Read the model definition and answer for the solid it produces. Units are mm, in the model's axes. A direction names the side the tool comes from. Round coordinates to 2 decimals unless told otherwise and drop trailing zeros. Order: outer loops, then holes, each group sorted by start corner. A loop starts at its lowest first (then second) coordinate and runs counter-clockwise, first axis right, second up. Notation, with made-up numbers: (19, 11.25) -> (27, 11.25) arc R14 cw to (27, 19.25) -> close; hole circle Ø10 at (35.5, 2). An arc over 180 degrees is marked (long way). Use a Markdown table: item, result. Add a question column.
1. Section C-C, the plane x = 0 is taken. Give the vertices of the cut face in (y, z), then the cut area to 3 significant figures.
2. Given pin 1 (5.5 mm diameter, centred on x = 0, z = 0, fed in from -Y); pin 2 (2 mm diameter, centred on y = -5.5, z = -2.5, fed in from +X); pin 3 (5 mm diameter, centred on y = -3.5, z = 1, fed in from -X), each flat-ended and moving along its own axis, determine where each tip first touches the part or whether it passes through.
3. For faces 5 (the face through (0, 1.2, 0)), 6 (the face through (9.224, 0.493, -9.331)), 7 (the face through (11.04, 2.46, -10.91)), determine the directions among +Z, -Z, +X, -X, +Y, -Y from which every point of the face is accessible in a straight line to the end or side of a thin tool.
4. Section D-D, the plane x = -11 is taken. Give the vertices of the cut face in (y, z), then the cut area to 3 significant figures.
5. Section A-A, the plane y = 4.25 is taken. Give the vertices of the cut face in (x, z).
6. Section B-B, the plane z = 0 is taken. Give the vertices of the cut face in (x, y), then the cut area to 3 significant figures.
7. Consider L1, parallel to X at y = 0.75, z = -1; L2, parallel to X at y = -5.5, z = 0; L3, parallel to Z at x = 10.5, y = 0.5. Determine where each line is inside the solid, lowest interval first. Write a range as [from, to].
8. The mould has two halves that part along Z. Classify faces 1 (the face through (6, 0, 0)), 2 (the face through (-10.91, 2.46, -11.04)), 3 (the face through (0.1, 0.5, 14.32)), 4 (the face through (0, 2, 15.52)): +Z half, -Z half, draft (parallel to the pull), parting line (faces both ways), or undercut.
```python
from build123d import *

# Parameters (mm, degrees)
EXTRUDE_1_DEPTH     = 5
CUT_EXTRUDE_1_DEPTH = 1
SKETCH_6_R          = 6.15
CUT_EXTRUDE_2_DEPTH = 3.8
SKETCH_8_R          = 4.15
SKETCH_8_R_2        = 3.15
EXTRUDE_4_DEPTH     = 7
SKETCH_9_R          = 5
SKETCH_9_R_2        = 4.15
EXTRUDE_5_DEPTH     = 2


with BuildPart() as part:
    # 스케치1 → 보스-돌출1 (new body)
    with BuildSketch(Plane(origin=(0, 0, 0), x_dir=(1, 0, 0), z_dir=(0, 1, 0))):
        Polygon((15.520132754, 6.428649477), (6.428649477, 15.520132754), (-6.428649477, 15.520132754), (-15.520132754, 6.428649477), (-15.520132754, -6.428649477), (-6.428649477, -15.520132754), (6.428649477, -15.520132754), (15.520132754, -6.428649477), align=None)
        Polygon((5.931593202, 14.320132754), (-5.931593202, 14.320132754), (-14.320132754, 5.931593202), (-14.320132754, -5.931593202), (-5.931593202, -14.320132754), (5.931593202, -14.320132754), (14.320132754, -5.931593202), (14.320132754, 5.931593202), align=None, mode=Mode.SUBTRACT)
        Polygon((14.320132754, 5.931593202), (5.931593202, 14.320132754), (-5.931593202, 14.320132754), (-14.320132754, 5.931593202), (-14.320132754, -5.931593202), (-5.931593202, -14.320132754), (5.931593202, -14.320132754), (14.320132754, -5.931593202), align=None)
    extrude(amount=EXTRUDE_1_DEPTH)

    # 스케치3 → 컷-돌출1 (cut)
    with BuildSketch(Plane.XZ):
        Polygon((5.931593202, -14.320132754), (14.320132754, -5.931593202), (14.320132754, 5.931593202), (5.931593202, 14.320132754), (-5.931593202, 14.320132754), (-14.320132754, 5.931593202), (-14.320132754, -5.931593202), (-5.931593202, -14.320132754), align=None)
        Polygon((5.434536927, -13.120132754), (13.120132754, -5.434536927), (13.120132754, 5.434536927), (5.434536927, 13.120132754), (-5.434536927, 13.120132754), (-13.120132754, 5.434536927), (-13.120132754, -5.434536927), (-5.434536927, -13.120132754), align=None, mode=Mode.SUBTRACT)
    extrude(amount=-CUT_EXTRUDE_1_DEPTH, mode=Mode.SUBTRACT)

    # 스케치6 → 컷-돌출2 (cut)
    with BuildSketch(Plane(origin=(0, 5, 0), x_dir=(1, 0, 0), z_dir=(0, 1, 0))):
        with Locations(Location((0, 0, 0), (0, 0, 270))):
            Circle(SKETCH_6_R)
    extrude(amount=-CUT_EXTRUDE_2_DEPTH, mode=Mode.SUBTRACT)

    # 스케치8 → 보스-돌출4 (add)
    with BuildSketch(Plane.XZ):
        with Locations(Location((0, 0, 0), (0, 0, 90))):
            Circle(SKETCH_8_R)
        with Locations(Location((0, 0, 0), (0, 0, 270))):
            Circle(SKETCH_8_R_2, mode=Mode.SUBTRACT)
    extrude(amount=EXTRUDE_4_DEPTH)

    # 스케치9 → 보스-돌출5 (add)
    with BuildSketch(Plane.XZ):
        with Locations(Location((0, 0, 0), (0, 0, 90))):
            Circle(SKETCH_9_R)
        with Locations(Location((0, 0, 0), (0, 0, 270))):
            Circle(SKETCH_9_R_2, mode=Mode.SUBTRACT)
    extrude(amount=EXTRUDE_5_DEPTH)


solid = part.part
```
Verdict:
| question | item | result |
|---|---|---|
| 1 | outline | (-7, -4.15) -> (-2, -4.15) -> (-2, -5) -> (0, -5) -> (0, -13.12) -> (1, -13.12) -> (1, -14.32) -> (0, -14.32) -> (0, -15.52) -> (5, -15.52) -> (5, -6.15) -> (1.2, -6.15) -> (1.2, 6.15) -> (5, 6.15) -> (5, 15.52) -> (0, 15.52) -> (0, 14.32) -> (1, 14.32) -> (1, 13.12) -> (0, 13.12) -> (0, 5) -> (-2, 5) -> (-2, 4.15) -> (-7, 4.15) -> (-7, 3.15) -> (0, 3.15) -> (0, -3.15) -> (-7, -3.15) -> close |
| 1 | area | 123 mm2 |
| 2 | pin 1 | stops at y = 0 |
| 2 | pin 2 | stops at x = 3.87 |
| 2 | pin 3 | stops at x = -5 |
| 3 | face 5 | +Y |
| 3 | face 6 | -Y |
| 3 | face 7 | -Z, +X, +Y, -Y |
| 4 | outline | (0, -10.95) -> (5, -10.95) -> (5, 10.95) -> (0, 10.95) -> (0, 9.25) -> (1, 9.25) -> (1, 7.55) -> (0, 7.55) -> (0, -7.55) -> (1, -7.55) -> (1, -9.25) -> (0, -9.25) -> close |
| 4 | area | 106 mm2 |
| 5 | outline | (-15.52, -6.43) -> (-6.43, -15.52) -> (6.43, -15.52) -> (15.52, -6.43) -> (15.52, 6.43) -> (6.43, 15.52) -> (-6.43, 15.52) -> (-15.52, 6.43) -> close; hole circle Ø12.3 at (0, 0) |
| 6 | outline | (-15.52, 0) -> (-14.32, 0) -> (-14.32, 1) -> (-13.12, 1) -> (-13.12, 0) -> (-5, 0) -> (-5, -2) -> (-4.15, -2) -> (-4.15, -7) -> (-3.15, -7) -> (-3.15, 0) -> (3.15, 0) -> (3.15, -7) -> (4.15, -7) -> (4.15, -2) -> (5, -2) -> (5, 0) -> (13.12, 0) -> (13.12, 1) -> (14.32, 1) -> (14.32, 0) -> (15.52, 0) -> (15.52, 5) -> (6.15, 5) -> (6.15, 1.2) -> (-6.15, 1.2) -> (-6.15, 5) -> (-15.52, 5) -> close |
| 6 | area | 123 mm2 |
| 7 | L1 | x = [-15.52, -14.32], [-13.12, 13.12], [14.32, 15.52] |
| 7 | L2 | x = [-4.15, -3.15], [3.15, 4.15] |
| 7 | L3 | z = [-11.45, -9.75], [-8.05, 8.05], [9.75, 11.45] |
| 8 | face 1 | draft |
| 8 | face 2 | -Z half |
| 8 | face 3 | undercut |
| 8 | face 4 | +Z half |
